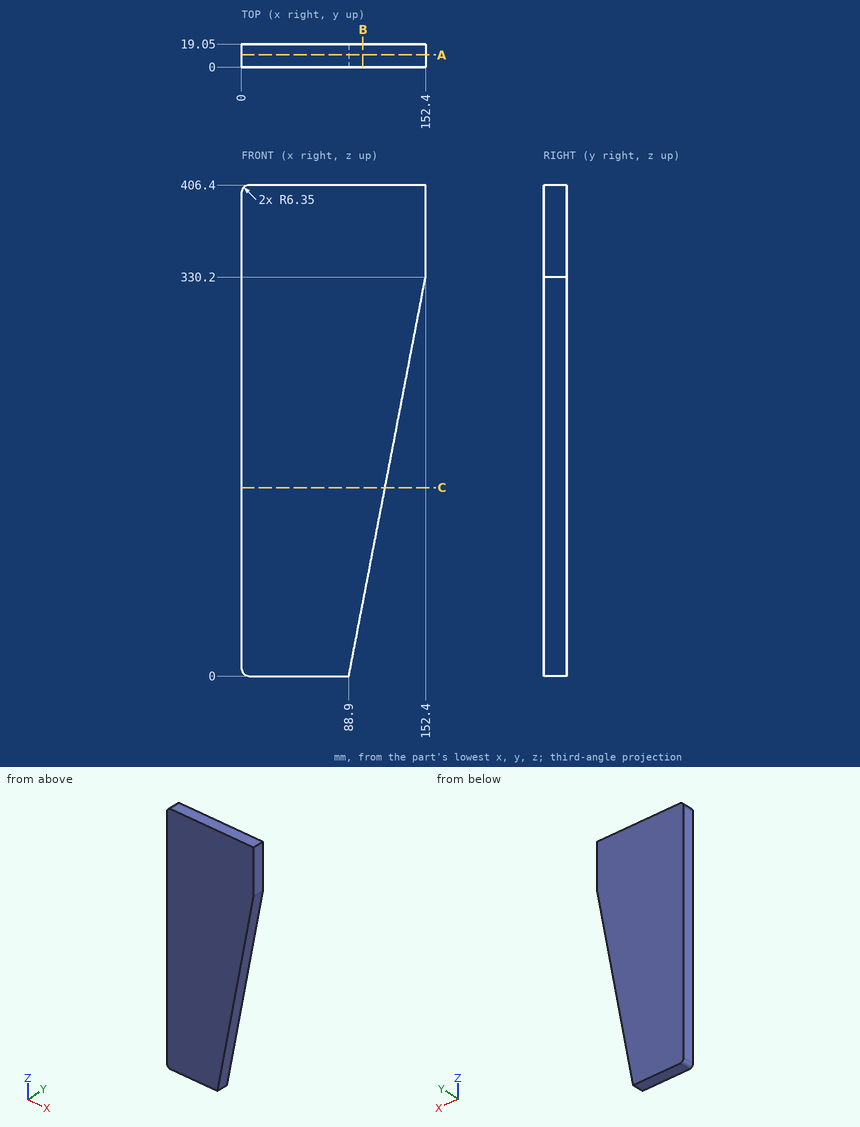
Check sheet for the drawn part. Datum: minimum x, y, z corner. Units: mm. Round coordinates to 2 decimals unless told otherwise and drop trailing zeros. Order: outer loops, then holes, each group sorted by start corner. A loop starts at its lowest first (then second) coordinate and runs counter-clockwise, first axis right, second up.
1) Section check A-A (y = 10). Record the boundary of the cut face in (x, z).
2) Section check B-B (x = 100.5). Record the boundary of the cut face in (y, z), and give its area (3 significant figures).
3) Go/stop test with flat-tipped pins: pin 1 Ø5 at (y, z) = (16.5, 136) entering from +X; pin 2 Ø2 at (y, z) = (7.5, 70) entering from +X. Record where each tip stops, or that it passes through.
4) Scan lines: line 1 (X direction, y = 10, z = 151); line 2 (X direction, y = 9.75, z = 244.5). Record each from-to range of solid material in increasing order.
5) Section check C-C (z = 156). Record the boundary of the cut face in (x, y), and give its area (3 significant figures).
Result:
1. outline: (0, 6.35) arc R6.35 ccw to (6.35, 0) - (88.9, 0) - (152.4, 330.2) - (152.4, 406.4) - (6.35, 406.4) arc R6.35 ccw to (0, 400.05) - close
2. outline: (0, 60.32) - (19.05, 60.32) - (19.05, 406.4) - (0, 406.4) - close
2. area: 6,590 mm2
3. pin 1: stops at x = 115.53
3. pin 2: stops at x = 102.55
4. line 1: x = 0 to 117.94
4. line 2: x = 0 to 135.92
5. outline: (0, 0) - (118.9, 0) - (118.9, 19.05) - (0, 19.05) - close
5. area: 2,270 mm2
